from build123d import *

# Parameters (mm, degrees)
BOSS_EXTRUDE1_DEPTH = 5
SKETCH2_R           = 1.5
CUT_EXTRUDE1_DEPTH  = 10
SKETCH3_R           = 2.5
CUT_EXTRUDE2_DEPTH  = 10
CIRPATTERN1_COUNT   = 3


with BuildPart() as part:
    # Sketch1 → Boss-Extrude1 (new, symmetric)
    with BuildSketch(Plane.XY):
        Polygon((86.602540378, 0), (43.301270189, 75), (-43.301270189, 75), (-86.602540378, 0), (-43.301270189, -75), (43.301270189, -75), align=None)
    extrude(amount=BOSS_EXTRUDE1_DEPTH, both=True)

    # Sketch2 → Cut-Extrude1 (cut)
    with BuildSketch(Plane.XZ.offset(75)):
        with Locations(Location((-10, 0, 0), (0, 0, 270))):
            Circle(SKETCH2_R)
        with Locations(Location((10, 0, 0), (0, 0, 270))):
            Circle(SKETCH2_R)
    cut_extrude1 = extrude(amount=-CUT_EXTRUDE1_DEPTH, mode=Mode.SUBTRACT)

    # Sketch3 → Cut-Extrude2 (cut)
    with BuildSketch(Plane.XY.offset(5)):
        Circle(SKETCH3_R)
    extrude(amount=-CUT_EXTRUDE2_DEPTH, mode=Mode.SUBTRACT)

    # CirPattern1: Cut-Extrude1 ×3 about axis
    cirpattern1_axis = Axis((0, 0, 0), (0, 0, 1))
    for i in range(1, CIRPATTERN1_COUNT):
        add(cut_extrude1.rotate(cirpattern1_axis, i * 360 / CIRPATTERN1_COUNT), mode=Mode.SUBTRACT)


solid = part.part
Input: part model. Units: mm. Frame: model coordinates. Round coordinates to 2 decimals unless told otherwise and drop trailing zeros. Write each loop counter-clockwise with the first axis right and the second up, starting at its lowest first coordinate (ties: lowest second). Pieces come first, ordered by that corner, then holes.
1) Cut plane B-B (z = 3). Return the cut outline in (x, y).
2) Cut plane C-C (y = 56). Return the cut outline in (x, z).
3) Cut plane D-D (y = -59). Return the cut outline in (x, z), then the cut area to 3 significant figures.
4) Draft query along Y for faces 1 (the flat face through (-64.65, 38.02, 0.07)), 2 (the flat face through (18, 1, 5)), 3 (the cylindrical face through (-0.54, -2.44, 0.07)). Return one class per face: pulls with the +Y half, pulls with the -Y half, needs draft (parallel to the pull), parting line crosses it, or undercut.
5) Contact query for flat-ended pins moving along their axis: P1, Ø1, axis at x = 47.5, z = 3, coming from the -Y side; P2, Ø1, axis at x = -67.5, z = -0.5, coming from the -Y side; P3, Ø1.5, axis at y = 20, z = 3, coming from the -X side. Output: stop coordinate, or through.
6) Ray query, L1, parallel to X at y = -71.75, z = 0; L2, parallel to X at y = -68, z = 0; L3, parallel to Y at x = -67, z = 0. Return the intervals inside material, ascending.
7) Cut plane A-A (x = 0). Return the cut outline in (y, z), then the cut area to 3 significant figures.
Geometry says:
1. outline: (-86.6, 0) - (-43.3, -75) - (43.3, -75) - (86.6, 0) - (43.3, 75) - (-43.3, 75) - close; hole circle Ø5 at (0, 0)
2. outline: (-54.27, -5) - (54.27, -5) - (54.27, 5) - (-54.27, 5) - close
3. outline: (-52.54, -5) - (52.54, -5) - (52.54, 5) - (-52.54, 5) - close
3. area: 1,050 mm2
4. face 1: pulls with the +Y half
4. face 2: needs draft
4. face 3: undercut
5. P1: stops at y = -68.59
5. P2: stops at y = -33.95
5. P3: stops at x = -75.49
6. L1: x = -45.18 to -11.5, -8.5 to 8.5, 11.5 to 45.18
6. L2: x = -47.34 to -11.5, -8.5 to 8.5, 11.5 to 47.34
6. L3: y = -33.95 to 25.4, 28.87 to 33.95
7. outline: (-75, -5) - (-2.5, -5) - (-2.5, 5) - (-75, 5) - close; (2.5, -5) - (75, -5) - (75, 5) - (2.5, 5) - close
7. area: 1,450 mm2
